Verification items for the finished model (mm, model axes). Face numbers are marked on the shaded views. A direction names the side the tool comes from. Give positions to 0.01 mm unless a question says otherwise; leave off trailing zeros. Order: outer loops, then holes, each group sorted by start corner. A loop starts at its lowest first (then second) coordinate and runs counter-clockwise, first axis right, second up. Notation, with made-up numbers: (58, 73) -> (103, 73) arc R21 cw to (103, 84) -> close; hole circle Ø4 at (8.25, 82). An arc over 180 degrees is marked (long way). One line per question, with ' | ' between items. Start each with the question number.
Q1. Go/stop test with flat-tipped pins: pin 1 (10 mm diameter, centred on x = -34, z = -16.5, fed in from +Y); pin 2 (3 mm diameter, centred on y = -12, z = 31.5, fed in from -X); pin 3 (1.5 mm diameter, centred on x = -70.5, z = -18.5, fed in from +Y). Record where each tip stops, or that it passes through.
Q2. Section check A-A on y = 0. Record the cut outline in (x, z), plus the area to 3 significant figures.
Q3. Section check D-D on x = -118. Record the cut outline in (y, z).
Q4. Access from +Z, -Z, +X, -X, +Y, -Y to the whole of each face (thin tool, end or side, straight path). Record for the marked faces 1, 2 and 3.
Q5. Material ranges on probe 1 along X at (y, z) = (14, -31.5); probe 2 along X at (y, z) = (19, -17); probe 3 along Y at (x, z) = (12, -2), recorded low to high. Write a range as [from, to].
Q6. Section check C-C on x = -2.5. Record the cut outline in (y, z).
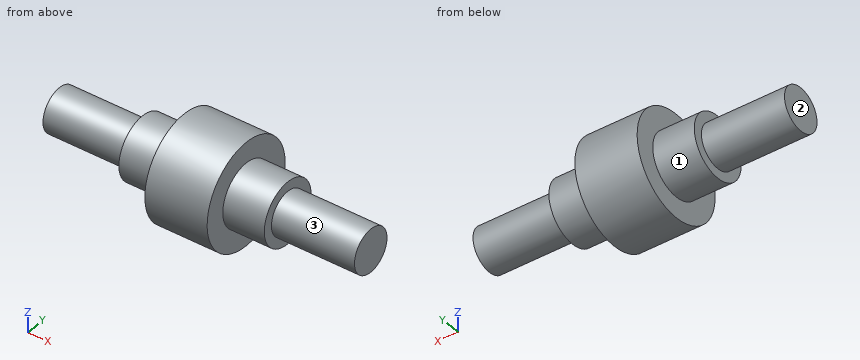
from build123d import *


with BuildPart() as part:
    # Sketch1 → Revolve6 (revolve)
    with BuildSketch(Plane.XY, mode=Mode.PRIVATE) as revolve6_sk:
        Polygon((-30, -50), (30, -50), (30, -30), (70, -30), (70, -20.825600731), (150, -20.825600731), (150, 0), (-150, 0), (-150, -20.825600731), (-70, -20.825600731), (-70, -30), (-30, -30), align=None)
    revolve(revolve6_sk.sketch.rotate(Axis((0, 0, 0), (-1, 0, 0)), 270), axis=Axis((0, 0, 0), (-1, 0, 0)))  # turned: the seam where the file's is


solid = part.part
Filled in:
1) pin 1: y = 48.14 | pin 2: x = -30 | pin 3: y = 24.04
2) outline: (-150, -20.83) -> (-70, -20.83) -> (-70, -30) -> (-30, -30) -> (-30, -50) -> (30, -50) -> (30, -30) -> (70, -30) -> (70, -20.83) -> (150, -20.83) -> (150, 20.83) -> (70, 20.83) -> (70, 30) -> (30, 30) -> (30, 50) -> (-30, 50) -> (-30, 30) -> (-70, 30) -> (-70, 20.83) -> (-150, 20.83) -> close | area: 17,500 mm²
3) outline: circle Ø41.65 at (0, 0)
4) face 1: -X | face 2: +Z, -Z, -X, +Y, -Y | face 3: +X
5) probe 1: [-30, 30] | probe 2: [-70, 70] | probe 3: [-49.96, 49.96]
6) outline: circle Ø100 at (0, 0)
